```python
from build123d import *

# Parameters (mm, degrees)
SKETCH1_R           = 0.423839805
SKETCH1_R_2         = 1.499879549
SKETCH1_R_3         = 0.508
BOSS_EXTRUDE1_DEPTH = 1.85


with BuildPart() as part:
    # Sketch1 → Boss-Extrude1 (new body)
    with BuildSketch(Plane.XY):
        with BuildLine():
            ThreePointArc((-7.175495363, -13.940801921), (-7.119699204, -14.075505763), (-6.984995363, -14.131301921))
            Line((-6.984995363, -14.131301921), (6.985004637, -14.131301921))
            ThreePointArc((6.985004637, -14.131301921), (7.099326594, -14.093185451), (7.1679, -13.994089221))
            Line((7.1679, -13.994089221), (7.1679, 11.913928619))
            ThreePointArc((7.1679, 11.913928619), (7.173590429, 11.94029461), (7.1755, 11.9672))
            Line((7.1755, 11.9672), (7.1755, 13.9992))
            ThreePointArc((7.1755, 13.9992), (7.119703561, 14.133900844), (6.985001921, 14.189695363))
            Line((6.985001921, 14.189695363), (-3.936998079, 14.189695363))
            ThreePointArc((-3.936998079, 14.189695363), (-4.009898233, 14.17519462), (-4.0717, 14.1339))
            Line((-4.0717, 14.1339), (-7.1197, 11.0859))
            ThreePointArc((-7.1197, 11.0859), (-7.16099462, 11.024098233), (-7.175495363, 10.951198079))
            Line((-7.175495363, 10.951198079), (-7.175495363, -13.940801921))
        make_face()
        with Locations((-6.223, -12.1628)):
            Circle(SKETCH1_R, mode=Mode.SUBTRACT)
        with Locations((-4.953, -12.1628)):
            Circle(SKETCH1_R, mode=Mode.SUBTRACT)
        with Locations((-2.413, -12.1628)):
            Circle(SKETCH1_R, mode=Mode.SUBTRACT)
        with Locations((-1.143, -12.1628)):
            Circle(SKETCH1_R, mode=Mode.SUBTRACT)
        with Locations((3.97765, -6.999)):
            Circle(SKETCH1_R_2, mode=Mode.SUBTRACT)
        with Locations((4.416979549, 3.001)):
            Circle(SKETCH1_R_2, mode=Mode.SUBTRACT)
        with Locations((-2.667, 8.6652)):
            Circle(SKETCH1_R_3, mode=Mode.SUBTRACT)
        with Locations((-0.127, 8.6652)):
            Circle(SKETCH1_R_3, mode=Mode.SUBTRACT)
        with Locations((2.413, 8.6652)):
            Circle(SKETCH1_R_3, mode=Mode.SUBTRACT)
        with Locations((4.953, 8.6652)):
            Circle(SKETCH1_R_3, mode=Mode.SUBTRACT)
    extrude(amount=BOSS_EXTRUDE1_DEPTH)


solid = part.part
```
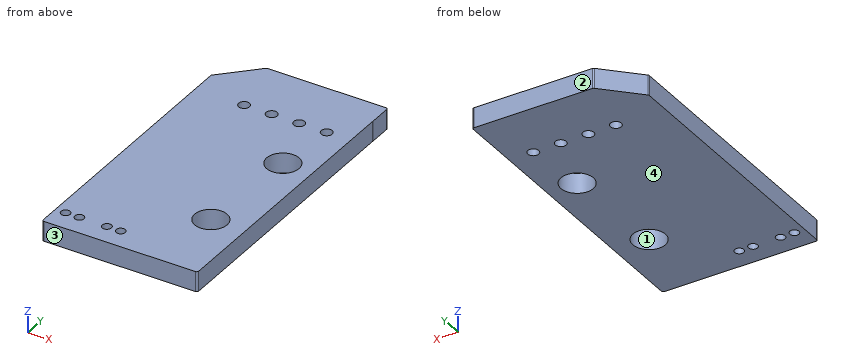
Build history of the part. All positions in model axes, mm. Face numbers are marked on the shaded views. Coordinates: 2 decimals unless noted, no trailing zeros. Order: outer loops, then holes, each group sorted by start corner. A loop starts at its lowest first (then second) coordinate and runs counter-clockwise, first axis right, second up. Notation, with made-up numbers: (47.5, -27) -> (98.5, -27) arc R27 ccw to (98.5, -10) -> close; hole circle Ø10 at (79, -8). An arc over 180 degrees is marked (long way). Answer in a Markdown table with one row per item. Add a question column.
Q1. Wall check: line 1 along Y through (x, z) = (4.25, 1); line 2 along Y through (x, z) = (4, 1.45); line 3 along X through (y, z) = (5.25, 1.45). Give the ranges that are in metal, low to high. Write a range as [from, to].
Q2. Band-saw the part on C-C, the plane z = 1.25. Give the number of separate pieces and of enclosed holes in the cut face, then the cut area to 3 significant figures.
Q3. Band-saw the part on A-A, the plane y = -8. List the corners of the cut face in (x, z), then the cut area to 3 significant figures.
Q4. Band-saw the part on B-B, the plane x = 4.75. List the corners of the cut face in (y, z), then the cut area to 3 significant figures.
Q5. Mould opens along Y. For the marked faces 1, 2, 3 and 4 say: +Y half, -Y half, draft (parallel to the pull), parting line (faces both ways), or undercut.
Q6. Drop flat-ended pins along their axis: pin 1 (0.9 mm diameter, centred on y = -3, z = 1, fed in from +X); pin 2 (2.5 mm diameter, centred on x = 4.42, y = 3, fed in from +Z). Give the stop position or say it passes through.
Answers follow:
| question | item | result |
|---|---|---|
| 1 | line 1 | [-14.13, -8.47], [-5.52, 1.51], [4.49, 14.19] |
| 1 | line 2 | [-14.13, -8.5], [-5.5, 1.56], [4.44, 14.19] |
| 1 | line 3 | [-7.18, 7.17] |
| 2 | separate pieces | 1 |
| 2 | enclosed holes | 10 |
| 2 | area | 382 mm^2 |
| 3 | outline | (-7.18, 0) -> (2.86, 0) -> (2.86, 1.85) -> (-7.18, 1.85) -> close; (5.09, 0) -> (7.17, 0) -> (7.17, 1.85) -> (5.09, 1.85) -> close |
| 3 | area | 22.4 mm^2 |
| 4 | outline | (-14.13, 0) -> (-8.28, 0) -> (-8.28, 1.85) -> (-14.13, 1.85) -> close; (-5.71, 0) -> (1.54, 0) -> (1.54, 1.85) -> (-5.71, 1.85) -> close; (4.46, 0) -> (8.2, 0) -> (8.2, 1.85) -> (4.46, 1.85) -> close; (9.13, 0) -> (14.19, 0) -> (14.19, 1.85) -> (9.13, 1.85) -> close |
| 4 | area | 40.5 mm^2 |
| 5 | face 1 | undercut |
| 5 | face 2 | +Y half |
| 5 | face 3 | -Y half |
| 5 | face 4 | draft |
| 6 | pin 1 | x = 7.17 |
| 6 | pin 2 | through |
